Model file for the job. Use its own axes, mm. A direction names the side the tool comes from. Coordinates: 2 decimals unless noted, no trailing zeros. Order: outer loops, then holes, each group sorted by start corner. A loop starts at its lowest first (then second) coordinate and runs counter-clockwise, first axis right, second up. Notation, with made-up numbers: (-19.5, 63.5) -> (18.5, 63.5) arc R17 cw to (18.5, 68.5) -> close; hole circle Ø4 at (44, 39). An arc over 180 degrees is marked (long way). Return JSON: item names as keys, results as strings. Group by question number.
1) Cut at B-B (z = 0.6). Write the cut outline in (x, y), and give its area (3 significant figures).
2) Flat gauge pin, fed straight in: pin 1 (4.5 mm diameter, centred on x = -42, y = 27, fed in from -Z). Where does the tip first touch, or does it go through?
3) Which spindle directions (+Z, -Z, +X, -X, +Y, -Y) get a long thin tool onto all of the face, cutting with end or side? Do faces 1 (the cylindrical face through (-55.9, 16.6, 1.6)), 2 (the flat face through (1, 32, 2)). Say none if no direction does.
4) Cut at C-C (x = -56). Write the cut outline in (y, z) (3 decimals), and give its area (3 significant figures).
5) Pull direction Y, two halves, no side cores. Call faces 3 (the flat face through (53.4, 10, 2)), 4 (the flat face through (-1, 16, 3.175)), 5 (the flat face through (-53.4, 10, 2)), 6 (the flat face through (-55, 27, 2)): +Y half, -Y half, draft (parallel to the pull), parting line (faces both ways), or undercut.
6) Probe line 1 (X direction, y = 9.5, z = 0.4); line 2 (Y direction, x = 42, z = 0.3); line 3 (Y direction, x = 39.5, z = 2.9). List the from-to ranges inside material, lowest first.
7) Cut at D-D (x = 42). Write the cut outline in (y, z) (3 decimals), and give its area (3 significant figures).
8) Cut at A-A (y = 27). Write the cut outline in (x, z) (3 decimals), and give its area (3 significant figures).
from build123d import *

# Parameters (mm, degrees)
F0_W     = 60
F0_H     = 32
F1_DEPTH = 3.175
F2_R     = 1.65
F3_DEPTH = 3.176
F4_SIZE  = 2
F5_SIZE  = 10


with BuildPart() as f1:
    # F0 (on Top) → F1 (new body)
    with BuildSketch(Plane.XY):
        with Locations((-30, 16)):
            Rectangle(F0_W, F0_H)
        with Locations((30, 16)):
            Rectangle(F0_W, F0_H)
    extrude(amount=F1_DEPTH)

    # F2 (on face) → F3 (cut, through all)
    with BuildSketch(Plane.XY.offset(3.175)):
        with BuildLine():
            ThreePointArc((-58.6, 14), (-56, 11.4), (-53.4, 14))
            ThreePointArc((-53.4, 14), (-56, 16.6), (-58.6, 14))
        make_face()
        with Locations((-42, 27)):
            Circle(F2_R)
        with Locations((42, 27)):
            Circle(F2_R)
        with BuildLine():
            ThreePointArc((53.4, 14), (56, 11.4), (58.6, 14))
            ThreePointArc((58.6, 14), (56, 16.6), (53.4, 14))
        make_face()
        with BuildLine():
            Line((-53.4, 6), (-53.4, 14))
            ThreePointArc((-53.4, 14), (-56, 11.4), (-58.6, 14))
            Line((-58.6, 14), (-58.6, 6))
            ThreePointArc((-58.6, 6), (-56, 8.6), (-53.4, 6))
        make_face()
        with BuildLine():
            Line((-58.6, 6), (-53.4, 6))
            ThreePointArc((-53.4, 6), (-56, 8.6), (-58.6, 6))
        make_face()
        with BuildLine():
            ThreePointArc((-58.6, 6), (-56, 3.4), (-53.4, 6))
            Line((-53.4, 6), (-58.6, 6))
        make_face()
        with BuildLine():
            Line((58.6, 6), (58.6, 14))
            ThreePointArc((58.6, 14), (56, 11.4), (53.4, 14))
            Line((53.4, 14), (53.4, 6))
            ThreePointArc((53.4, 6), (56, 8.6), (58.6, 6))
        make_face()
        with BuildLine():
            Line((53.4, 6), (58.6, 6))
            ThreePointArc((58.6, 6), (56, 8.6), (53.4, 6))
        make_face()
        with BuildLine():
            ThreePointArc((53.4, 6), (56, 3.4), (58.6, 6))
            Line((58.6, 6), (53.4, 6))
        make_face()
    extrude(amount=-F3_DEPTH, mode=Mode.SUBTRACT)

    # F4
    f4_edges = [f1.edges().sort_by_distance(p)[0] for p in [
        (-43.65, 27, 3.175),
        (40.35, 27, 3.175),
    ]]
    chamfer(f4_edges, length=F4_SIZE)

    # F5
    f5_edges = [f1.edges().sort_by_distance(p)[0] for p in [
        (-60, 32, 1.5875),
        (60, 32, 1.5875),
    ]]
    chamfer(f5_edges, length=F5_SIZE)


solid = f1.part
Answers below:
{
 "1": {"outline": "(-60, 0) -> (60, 0) -> (60, 22) -> (50, 32) -> (-50, 32) -> (-60, 22) -> close; hole (-58.6, 6) arc R2.6 ccw to (-53.4, 6) -> (-53.4, 14) arc R2.6 ccw to (-58.6, 14) -> close; hole circle Ø3.3 at (-42, 27); hole circle Ø3.3 at (42, 27); hole (53.4, 6) arc R2.6 ccw to (58.6, 6) -> (58.6, 14) arc R2.6 ccw to (53.4, 14) -> close", "area": "3,600 mm^2"},
 "2": {"pin 1": "stops at z = 0"},
 "3": {"face 1": "+Z, -Z", "face 2": "+Z, -Z, +X, -X, +Y"},
 "4": {"outline": "(0, 0) -> (3.4, 0) -> (3.4, 3.175) -> (0, 3.175) -> close; (16.6, 0) -> (26, 0) -> (26, 3.175) -> (16.6, 3.175) -> close", "area": "40.6 mm^2"},
 "5": {"face 3": "undercut", "face 4": "draft", "face 5": "undercut", "face 6": "+Y half"},
 "6": {"line 1": "x = -60 to -58.6, -53.4 to 53.4, 58.6 to 60", "line 2": "y = 0 to 25.35, 28.65 to 32", "line 3": "y = 0 to 24.73, 29.27 to 32"},
 "7": {"outline": "(0, 0) -> (25.35, 0) -> (25.35, 1.175) -> (23.35, 3.175) -> (0, 3.175) -> close; (28.65, 0) -> (32, 0) -> (32, 3.175) -> (30.65, 3.175) -> (28.65, 1.175) -> close", "area": "87.1 mm^2"},
 "8": {"outline": "(-55, 0) -> (-43.65, 0) -> (-43.65, 1.175) -> (-45.65, 3.175) -> (-55, 3.175) -> close; (-40.35, 0) -> (40.35, 0) -> (40.35, 1.175) -> (38.35, 3.175) -> (-38.35, 3.175) -> (-40.35, 1.175) -> close; (43.65, 0) -> (55, 0) -> (55, 3.175) -> (45.65, 3.175) -> (43.65, 1.175) -> close", "area": "320 mm^2"}
}
